Part print with two shaded views. Sizes in mm from the minimum x, y, z corner. Round coordinates to 2 decimals unless told otherwise and drop trailing zeros. Order: outer loops, then holes, each group sorted by start corner. A loop starts at its lowest first (then second) coordinate and runs counter-clockwise, first axis right, second up. Notation, with made-up numbers: (6.5, 58.5) - (60.5, 58.5) arc R11 cw to (60.5, 63.5) - close; hole circle Ø2 at (23, 70). An arc over 180 degrees is marked (long way). Write item = value, one per line.
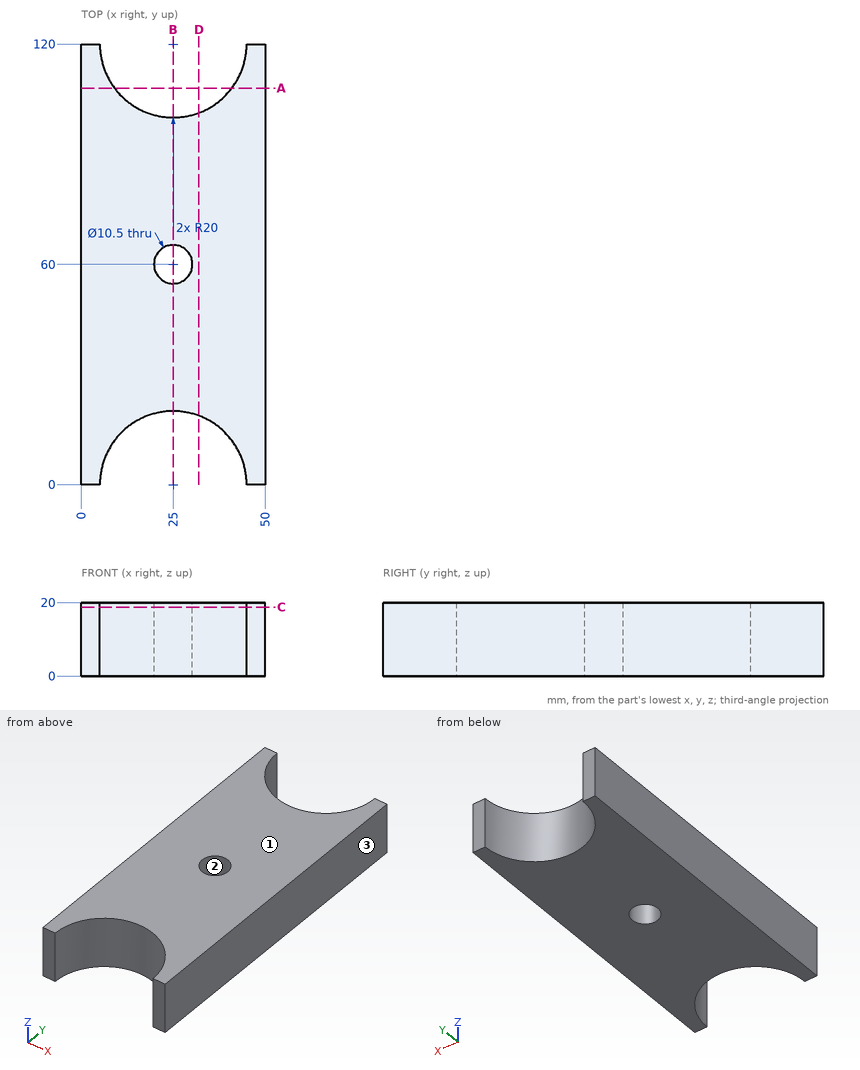
1) Cut at B-B (x = 25). Write the cut outline in (y, z).
Conclusion:
outline = (20, 0) - (54.75, 0) - (54.75, 20) - (20, 20) - close; (65.25, 0) - (100, 0) - (100, 20) - (65.25, 20) - close
2) Flat gauge pins, fed straight in: pin 1 Ø4 at (x, z) = (16.5, 14) entering from +Y; pin 2 Ø6 at (x, z) = (16, 12) entering from -Y. Where does each tip first touch, or does it go through?
Conclusion:
pin_1 = 102.98
pin_2 = 16
3) Cut at A-A (y = 108). Write the cut outline in (x, z), and give its area (3 significant figures).
Conclusion:
outline = (0, 0) - (9, 0) - (9, 20) - (0, 20) - close; (41, 0) - (50, 0) - (50, 20) - (41, 20) - close
area = 360 mm^2
4) Cut at C-C (z = 18.75). Write the cut outline in (x, y), and give its area (3 significant figures).
Conclusion:
outline = (0, 0) - (5, 0) arc R20 cw to (45, 0) - (50, 0) - (50, 120) - (45, 120) arc R20 cw to (5, 120) - (0, 120) - close; hole circle Ø10.5 at (25, 60)
area = 4,660 mm^2
5) Wall check: line 1 along Y through (x, z) = (25, 6); line 2 along X through (y, z) = (111, 9.5); line 3 along X through (y, z) = (115.5, 14.75). Give the ranges that are in metal, low to high.
Conclusion:
line_1 = 20 to 54.75, 65.25 to 100
line_2 = 0 to 7.14, 42.86 to 50
line_3 = 0 to 5.51, 44.49 to 50
6) Cut at D-D (x = 32). Write the cut outline in (y, z) (3 decimals).
Conclusion:
outline = (18.735, 0) - (101.265, 0) - (101.265, 20) - (18.735, 20) - close
7) Mould opens along X. For the marked faces 1, 2 and 3 say: +X half, -X half, draft (parallel to the pull), parting line (faces both ways), or undercut.
Conclusion:
face_1 = draft
face_2 = undercut
face_3 = +X half
